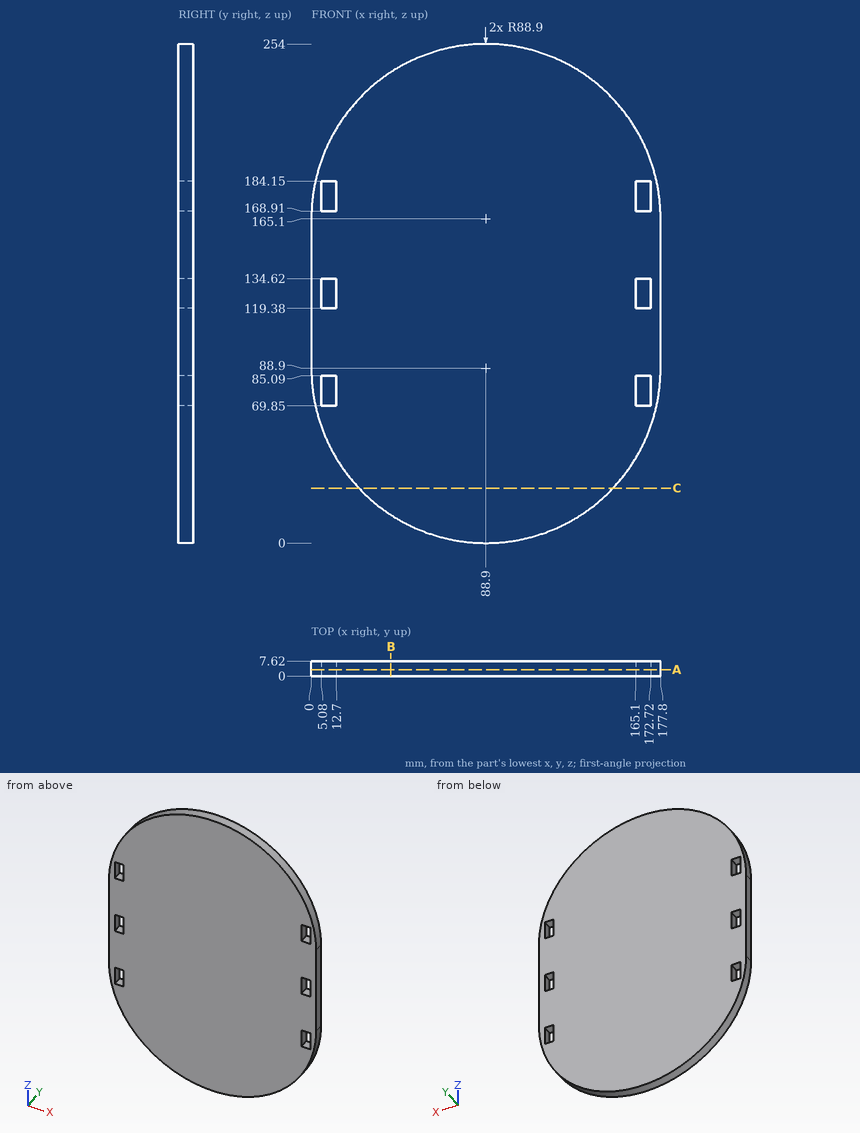
Study the drawing (mm; zero at the part's minimum x, y, z) and answer. Give positions to 0.01 mm unless a question says otherwise; leave off trailing zeros. Write each loop counter-clockwise with the first axis right and the second up, starting at its lowest first coordinate (ties: lowest second). Pieces come first, ordered by that corner, then holes. Notation, with made-up numbers: (-22, 87.25) - (10, 87.25) arc R11 cw to (10, 101.25) - close; hole circle Ø5 at (4.5, -21). An arc over 180 degrees is marked (long way). Write item = value, one per line. Start each with the question number.
Item 1: Find section B-B (x = 40.5). Give the vertices of the cut face in (y, z), then the cut area to 3 significant figures.
Item 2: Each of these flat-tipped pins is pushed along its axis until it touches: P1, Ø2, axis at y = 1.5, z = 26.5, coming from the -X side; P2, Ø4, axis at y = 4.5, z = 75.5, coming from the -X side; P3, Ø2.5, axis at y = 3.5, z = 178, coming from the -X side. Where does it stop, or does it pass through?
Item 3: Find the intervals of material crossed by probe 1 along X at (y, z) = (4.25, 127.5); probe 2 along Z at (x, y) = (169.5, 2.25); probe 3 along X at (y, z) = (4, 174), in increasing order. Write a range as [from, to].
Item 4: Find section A-A (y = 3.25). Give the vertices of the cut face in (x, z).
Item 5: Find section C-C (z = 28). Give the vertices of the cut face in (x, y), then the cut area to 3 significant figures.
Response:
q1.outline = (0, 14.33) - (7.62, 14.33) - (7.62, 239.67) - (0, 239.67) - close
q1.area = 1,720 mm²
q2.P1 = 24.61
q2.P2 = 0.73
q2.P3 = 0.77
q3.probe_1 = [0, 5.08], [12.7, 165.1], [172.72, 177.8]
q3.probe_2 = [51.39, 69.85], [85.09, 119.38], [134.62, 168.91], [184.15, 202.61]
q3.probe_3 = [0.45, 5.08], [12.7, 165.1], [172.72, 177.35]
q4.outline = (0, 88.9) arc R88.9 ccw to (177.8, 88.9) - (177.8, 165.1) arc R88.9 ccw to (0, 165.1) - close; hole (5.08, 69.85) - (12.7, 69.85) - (12.7, 85.09) - (5.08, 85.09) - close; hole (5.08, 119.38) - (12.7, 119.38) - (12.7, 134.62) - (5.08, 134.62) - close; hole (5.08, 168.91) - (12.7, 168.91) - (12.7, 184.15) - (5.08, 184.15) - close; hole (165.1, 69.85) - (172.72, 69.85) - (172.72, 85.09) - (165.1, 85.09) - close; hole (165.1, 119.38) - (172.72, 119.38) - (172.72, 134.62) - (165.1, 134.62) - close; hole (165.1, 168.91) - (172.72, 168.91) - (172.72, 184.15) - (165.1, 184.15) - close
q5.outline = (24.14, 0) - (153.66, 0) - (153.66, 7.62) - (24.14, 7.62) - close
q5.area = 987 mm²
